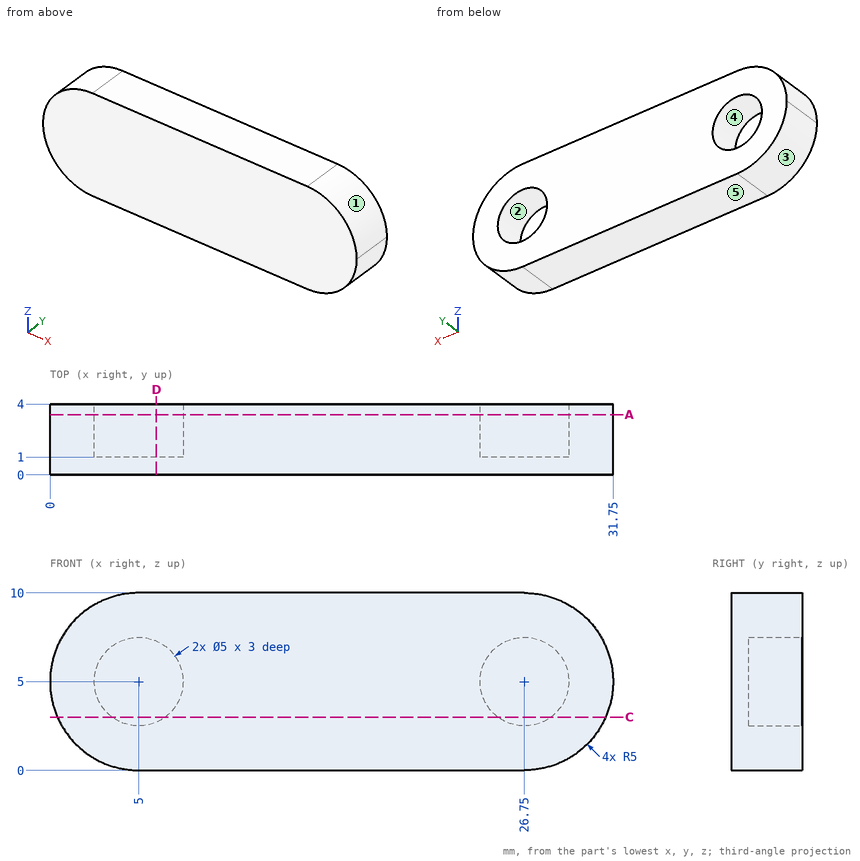
Here's the drawing with two shaded views (mm, measured from the low corner). I have some questions. A direction names the side the tool comes from. Give positions to 0.01 mm unless a question says otherwise; leave off trailing zeros. Order: outer loops, then holes, each group sorted by start corner. A loop starts at its lowest first (then second) coordinate and runs counter-clockwise, first axis right, second up. Notation, with made-up numbers: M 8.25,72 L 60.25,72 A29 ccw 60.25,101 Z; hole C -31.75,89.5 d6. An arc over 180 degrees is marked long. Answer as a JSON object with one key per item and string values. Group by question number.
1) We'd pull the mould along X, two halves only. Please class the marked faces 1, 2 and 3: pulls with the +X half, pulls with the -X half, needs draft (parallel to the pull), parting line crosses it, or undercut.
2) Suppose I cut it at D-D, the plane x = 6. Write out the boundary of the cut face in (y, z).
3) Please list where these lines run through material, in increasing order: L1, parallel to X at y = 2.65, z = 5; L2, parallel to Z at x = 26.75, y = 2.9; L3, parallel to X at y = 3.6, z = 4. Write a range as [from, to].
4) On a 3-axis mill with a long thin cutter (end or side, diameter ignored), from which of +Z, -Z, +X, -X, +Y, -Y can I reach the whole of each face in a straight line? I mean the marked faces 4 and 5. Say none if no direction works.
5) Suppose I cut it at A-A, the plane y = 3.4. Count the separate pieces of the cut face and the enclosed holes in it, plus the area to 3 significant figures.
6) Suppose I cut it at C-C, the plane z = 3. Write out the boundary of the cut face in (x, y), plus the area to 3 significant figures.
7) I'm going to push flat-ended pins straight in: pin 1 Ø1.5 at (x, z) = (27, 4.5) entering from +Y; pin 2 Ø1.5 at (y, z) = (1.5, 2) entering from -X (1 decimal); pin 3 Ø1.5 at (y, z) = (2.5, 2.5) entering from +X. Where does each tip first touch, or does it pass through?
Results found:
{
 "1": {"face 1": "pulls with the +X half", "face 2": "undercut", "face 3": "pulls with the -X half"},
 "2": {"outline": "M 0,0 L 4,0 L 4,2.71 L 1,2.71 L 1,7.29 L 4,7.29 L 4,10 L 0,10 Z"},
 "3": {"L1": "[0, 2.5], [7.5, 24.25], [29.25, 31.75]", "L2": "[0, 2.5], [7.5, 10]", "L3": "[0.1, 2.71], [7.29, 24.46], [29.04, 31.65]"},
 "4": {"face 4": "+Y", "face 5": "-Z, +X, -X, +Y, -Y"},
 "5": {"separate pieces": "1", "enclosed holes": "2", "area": "257 mm²"},
 "6": {"outline": "M 0.42,0 L 31.33,0 L 31.33,4 L 28.25,4 L 28.25,1 L 25.25,1 L 25.25,4 L 6.5,4 L 6.5,1 L 3.5,1 L 3.5,4 L 0.42,4 Z", "area": "106 mm²"},
 "7": {"pin 1": "y = 1", "pin 2": "x = 0.5", "pin 3": "x = 31.43"}
}
